```python
from build123d import *

# Parameters (mm, degrees)
SZKIC1_W                    = 125
SZKIC1_H                    = 80
DODANIE_WYCI_GNI_CIE1_DEPTH = 30
SKORUPA2_T                  = -3


with BuildPart() as part:
    # Szkic1 → Dodanie-wyciągnięcie1 (new body)
    with BuildSketch(Plane(origin=(0, 0, 0), x_dir=(1, 0, 0), z_dir=(0, 1, 0))):
        Rectangle(SZKIC1_W, SZKIC1_H)
    extrude(amount=-DODANIE_WYCI_GNI_CIE1_DEPTH)

    # Skorupa2
    skorupa2_openings = [part.faces().sort_by_distance(p)[0] for p in [
        (0, -30, 0),
    ]]
    offset(amount=SKORUPA2_T, openings=skorupa2_openings, kind=Kind.INTERSECTION)


solid = part.part
```
Build history of the part. All positions in model axes, mm. A direction names the side the tool comes from. Give positions to 0.01 mm unless a question says otherwise; leave off trailing zeros. Order: outer loops, then holes, each group sorted by start corner. A loop starts at its lowest first (then second) coordinate and runs counter-clockwise, first axis right, second up. Notation, with made-up numbers: M 48.25,-27 L 57.25,-27 A20 cw 57.25,-4 Z; hole C 20.5,65.25 d11. An arc over 180 degrees is marked long. Return JSON: item names as keys, results as strings.
Q1. Wall check: probe 1 along Z at (x, y) = (-40, -27); probe 2 along X at (y, z) = (-27.5, -8.5); probe 3 along Y at (x, z) = (-35.5, 5). Give the ranges that are in metal, low to high. Write a range as from..to.
Answer list:
{"probe 1": "z = -40..-37, 37..40", "probe 2": "x = -62.5..-59.5, 59.5..62.5", "probe 3": "y = -3..0"}
Q2. Flat gauge pin, fed straight in: pin 1 (1 mm diameter, centred on x = 47.5, z = 22, fed in from -Y). Where does the tip first touch, or does it go through?
Answer list:
{"pin 1": "stops at y = -3"}
Q3. Band-saw the part on A-A (y = -15.75). Give the cut face in (x, z), then the cut area to 3 significant figures.
Answer list:
{"outline": "M -62.5,-40 L 62.5,-40 L 62.5,40 L -62.5,40 Z; hole M -59.5,-37 L 59.5,-37 L 59.5,37 L -59.5,37 Z", "area": "1,190 mm^2"}
Q4. 3-axis set-ups, long thin cutter, end or side, ignore diameter. For faces 5 (the face through (-1, -15, -40)), 6 (the face through (-1, -16, 37)): which of +Z, -Z, +X, -X, +Y, -Y reach the whole face in a straight line?
Answer list:
{"face 5": "-Z, +X, -X, +Y, -Y", "face 6": "-Y"}
Q5. Band-saw the part on B-B (z = -28). Give the cut face in (x, y).
Answer list:
{"outline": "M -62.5,-30 L -59.5,-30 L -59.5,-3 L 59.5,-3 L 59.5,-30 L 62.5,-30 L 62.5,0 L -62.5,0 Z"}
Q6. Band-saw the part on C-C (x = 4.5). Give the cut face in (y, z), then the cut area to 3 significant figures.
Answer list:
{"outline": "M -30,-40 L 0,-40 L 0,40 L -30,40 L -30,37 L -3,37 L -3,-37 L -30,-37 Z", "area": "402 mm^2"}
Q7. Two-plate mould, pull along X, no slides. Class faces 1 (the face through (-1, 0, -1)), 2 (the face through (62.5, -15, 1)), 3 (the face through (-62.5, -15, 1)), 4 (the face through (59.5, -16, 1)): pulls with the +X half, pulls with the -X half, needs draft (parallel to the pull), parting line crosses it, or undercut.
Answer list:
{"face 1": "needs draft", "face 2": "pulls with the +X half", "face 3": "pulls with the -X half", "face 4": "undercut"}
